Part print with two shaded views. Sizes in mm from the minimum x, y, z corner. A direction names the side the tool comes from. Give positions to 0.01 mm unless a question says otherwise; leave off trailing zeros. Write each loop counter-clockwise with the first axis right and the second up, starting at its lowest first coordinate (ties: lowest second). Pieces come first, ordered by that corner, then holes. Notation, with made-up numbers: (0, 48) - (8, 48) arc R21 ccw to (8, 84) - close; hole circle Ø5 at (27.25, -31). An arc over 180 degrees is marked (long way). Answer as a JSON object with one key per item and string values. Group by question number.
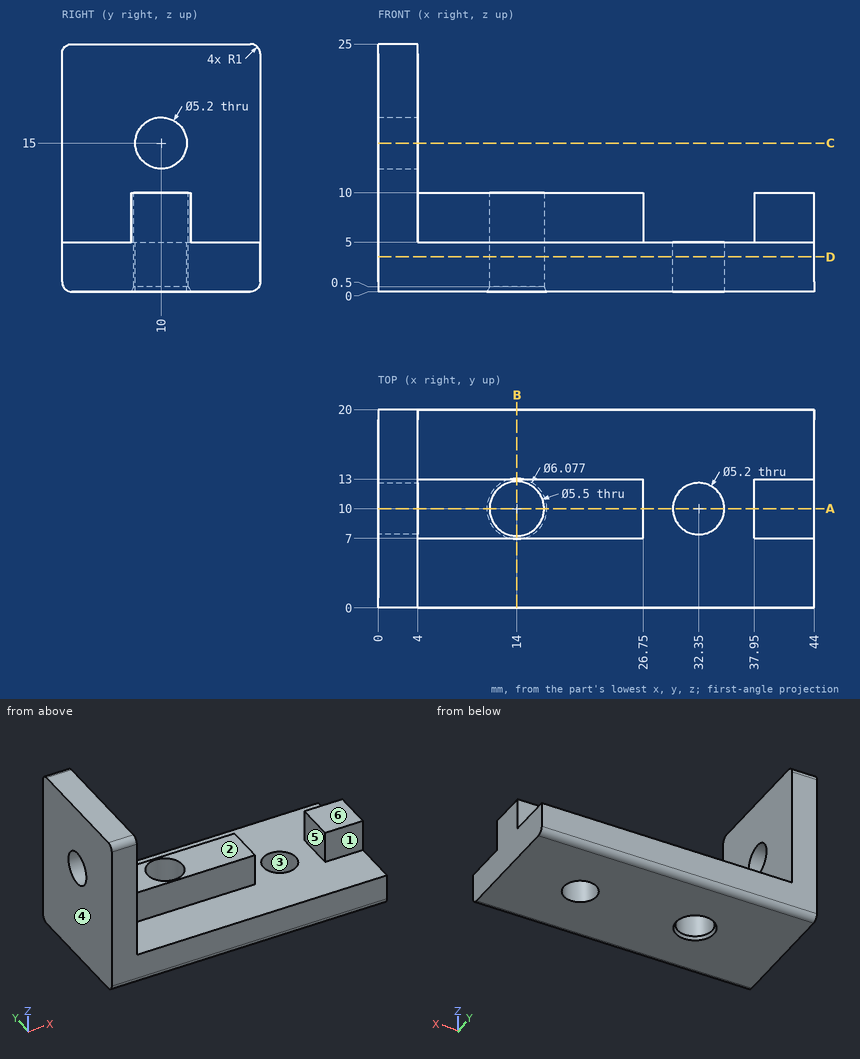
1) Saw through at C-C (z = 15). List the corners of the cut face in (x, y).
2) Saw through at B-B (x = 14). List the corners of the cut face in (y, z).
3) Saw through at A-A (y = 10). List the corners of the cut face in (x, z).
4) Drill centre lines: line 1 along Y through (x, z) = (32.5, 2) (1 decimal); line 2 along X through (y, z) = (15.75, 7); line 3 along Y through (x, z) = (14, 3). Where is each one in solid material? Low to high. Write a range as from..to.
5) Which spindle directions (+Z, -Z, +X, -X, +Y, -Y) get a long thin tool onto all of the face, cutting with end or side? Do the marked faces 1, 2 and 3. Say none if no direction does.
6) Two-plate mould, pull along X, no slides. Class the marked faces 4, 5 and 6: +X half, -X half, draft (parallel to the pull), parting line (faces both ways), or undercut.
7) Saw through at D-D (z = 3.5). List the corners of the cut face in (x, y), and give its area (3 significant figures).
8) Drop flat-ended pins along their axis: P1, Ø10, axis at x = 39, z = 14, coming from the -Y side; P2, Ø3, axis at x = 13, y = 11, coming from the +Z side; P3, Ø4, axis at y = 10, z = 15, coming from the -X side; P4, Ø1.5, axis at x = 33, y = 14, coming from the +Z side. Give the stop position or say it passes through.
Checks:
{
 "1": {"outline": "(0, 0) - (4, 0) - (4, 7.4) - (0, 7.4) - close; (0, 12.6) - (4, 12.6) - (4, 20) - (0, 20) - close"},
 "2": {"outline": "(0, 1) arc R1 ccw to (1, 0) - (6.96, 0) - (7.25, 0.5) - (7.25, 10) - (7, 10) - (7, 5) - (0, 5) - close; (12.75, 0.5) - (13.04, 0) - (19, 0) arc R1 ccw to (20, 1) - (20, 5) - (13, 5) - (13, 10) - (12.75, 10) - close"},
 "3": {"outline": "(0, 0) - (10.96, 0) - (11.25, 0.5) - (11.25, 10) - (4, 10) - (4, 12.4) - (0, 12.4) - close; (0, 17.6) - (4, 17.6) - (4, 25) - (0, 25) - close; (16.75, 0.5) - (17.04, 0) - (29.75, 0) - (29.75, 5) - (26.75, 5) - (26.75, 10) - (16.75, 10) - close; (34.95, 0) - (44, 0) - (44, 10) - (37.95, 10) - (37.95, 5) - (34.95, 5) - close"},
 "4": {"line 1": "0..7.4, 12.6..20", "line 2": "0..4", "line 3": "0..7.25, 12.75..20"},
 "5": {"face 1": "+Z, +X, -Y", "face 2": "+Z, +X, +Y, -Y", "face 3": "+Z, -Z"},
 "6": {"face 4": "-X half", "face 5": "undercut", "face 6": "draft"},
 "7": {"outline": "(0, 0) - (44, 0) - (44, 20) - (0, 20) - close; hole circle Ø5.5 at (14, 10); hole circle Ø5.2 at (32.35, 10)", "area": "835 mm2"},
 "8": {"P1": "y = 7", "P2": "z = 10", "P3": "through", "P4": "z = 5"}
}
